```python
from build123d import *

# Parameters (mm, degrees)
SKETCH1_R           = 35
BOSS_EXTRUDE1_DEPTH = 27.6
SKETCH2_R           = 40
BOSS_EXTRUDE2_DEPTH = 2.2
BOSS_EXTRUDE3_DEPTH = 4.4
FILLET3_R           = 2
SKETCH4_R           = 6.3
CUT_EXTRUDE1_DEPTH  = 34.2
SKETCH5_R           = 2.5
CUT_EXTRUDE2_DEPTH  = 4.4


with BuildPart() as part:
    # Sketch1 → Boss-Extrude1 (new body)
    with BuildSketch(Plane(origin=(0, 0, 0), x_dir=(1, 0, 0), z_dir=(0, 1, 0))):
        with Locations(Location((0, 0, 0), (0, 0, 90))):
            Circle(SKETCH1_R)
    extrude(amount=BOSS_EXTRUDE1_DEPTH)

    # Sketch2 → Boss-Extrude2 (add)
    with BuildSketch(Plane(origin=(0, 27.6, 0), x_dir=(1, 0, 0), z_dir=(0, 1, 0))):
        with Locations(Location((0, 0, 0), (0, 0, 270))):
            Circle(SKETCH2_R)
    extrude(amount=BOSS_EXTRUDE2_DEPTH)

    # Sketch3 → Boss-Extrude3 (add)
    with BuildSketch(Plane(origin=(0, 29.8, 0), x_dir=(1, 0, 0), z_dir=(0, 1, 0))):
        with BuildLine():
            Line((-25, 5), (-17.291616466, 5))
            ThreePointArc((-17.291616466, 5), (-12.727922061, 12.727922061), (-5, 17.291616466))
            Line((-5, 17.291616466), (-5, 25))
            Line((-5, 25), (5, 25))
            Line((5, 25), (5, 17.291616466))
            ThreePointArc((5, 17.291616466), (12.727922061, 12.727922061), (17.291616466, 5))
            Line((17.291616466, 5), (25, 5))
            Line((25, 5), (25, -5))
            Line((25, -5), (17.291616466, -5))
            ThreePointArc((17.291616466, -5), (12.727922061, -12.727922061), (5, -17.291616466))
            Line((5, -17.291616466), (5, -25))
            Line((5, -25), (-5, -25))
            Line((-5, -25), (-5, -17.291616466))
            ThreePointArc((-5, -17.291616466), (-12.727922061, -12.727922061), (-17.291616466, -5))
            Line((-17.291616466, -5), (-25, -5))
            Line((-25, -5), (-25, 5))
        make_face()
    extrude(amount=BOSS_EXTRUDE3_DEPTH)

    # Fillet3
    fillet3_edges = [part.edges().sort_by_distance(p)[0] for p in [
        (-25, 32, -5),
        (-25, 32, 5),
        (-17.291616466, 32, 5),
        (-5, 32, 17.291616466),
        (-5, 32, 25),
        (5, 32, 25),
        (5, 32, 17.291616466),
        (17.291616466, 32, 5),
        (25, 32, 5),
        (25, 32, -5),
        (17.291616466, 32, -5),
        (5, 32, -17.291616466),
        (5, 32, -25),
        (-5, 32, -25),
        (-5, 32, -17.291616466),
        (-17.291616466, 32, -5),
    ]]
    fillet(fillet3_edges, radius=FILLET3_R)

    # Sketch4 → Cut-Extrude1 (cut)
    with BuildSketch(Plane(origin=(0, 34.2, 0), x_dir=(1, 0, 0), z_dir=(0, 1, 0))):
        with Locations(Location((0, 0, 0), (0, 0, 270))):
            Circle(SKETCH4_R)
    extrude(amount=-CUT_EXTRUDE1_DEPTH, mode=Mode.SUBTRACT)

    # Sketch5 → Cut-Extrude2 (cut)
    with BuildSketch(Plane(origin=(0, 34.2, 0), x_dir=(1, 0, 0), z_dir=(0, 1, 0))):
        with Locations(Location((21, 0, 0), (0, 0, 270))):
            Circle(SKETCH5_R)
        with Locations(Location((0, -21, 0), (0, 0, 270))):
            Circle(SKETCH5_R)
        with Locations(Location((-21, 0, 0), (0, 0, 270))):
            Circle(SKETCH5_R)
        with Locations(Location((0, 21, 0), (0, 0, 270))):
            Circle(SKETCH5_R)
    extrude(amount=-CUT_EXTRUDE2_DEPTH, mode=Mode.SUBTRACT)


solid = part.part
```
The model under review builds one solid part; all positions refer to its coordinate system, in mm. A direction names the side the tool comes from. Give positions to 0.01 mm unless a question says otherwise; leave off trailing zeros. Write each loop counter-clockwise with the first axis right and the second up, starting at its lowest first coordinate (ties: lowest second). Pieces come first, ordered by that corner, then holes. Notation, with made-up numbers: (-6, -15.75) - (20, -15.75) arc R19 cw to (20, 3.25) - close; hole circle Ø9 at (45.25, 26). An arc over 180 degrees is marked (long way). Answer in a Markdown table with one row per item. Add a question column.
1. We need section B-B on z = -26. Write out the cut boundary in (x, y).
2. We need section A-A on x = 0. Write out the cut boundary in (y, z).
3. Tool access review of faces 1 (the flat face through (25, 32, 0)), 2 (the cylindrical face through (24.4, 32.03, 4.43)), 3 (the cylindrical face through (-4.43, 32.03, 24.4)), 4 (the cylindrical face through (-18.52, 32.03, -0.33)), 5 (the cylindrical face through (-24.43, 32.03, -4.4)): name each direction out of +Z, -Z, +X, -X, +Y, -Y from which nothing blocks a thin tool from reaching the whole face with its end or side.
4. We need section D-D on x = -8.5. Write out the cut boundary in (y, z), then the cut area to 3 significant figures.
5. We need section C-C on y = 31.5. State how many separate pieces and enclosed holes the cut face has, then the cut area to 3 significant figures.
6. Wall thickness on line 1 along X through (y, z) = (30.9, 0); line 2 along Y through (x, z) = (-25, -23); line 3 along X through (y, z) = (13.5, 0): over which ranges is each line inside the solid? List them lowest first. Write a range as [from, to].
7. Insertion check: P1, Ø12, axis at y = 9.5, z = -23.5, coming from the -X side; P2, Ø8, axis at y = 4.5, z = -12, coming from the -X side; P3, Ø2, axis at x = 20, y = 32, coming from the +Z side; P4, Ø11.5, axis at x = 0, z = 0, coming from the -Y side. Each pin has a flat end and moves straight along its axis. Give the tip position at first contact, or say it passes through.
Ans:
| question | item | result |
|---|---|---|
| 1 | outline | (-30.4, 27.6) - (-23.43, 27.6) - (-23.43, 0) - (23.43, 0) - (23.43, 27.6) - (30.4, 27.6) - (30.4, 29.8) - (-30.4, 29.8) - close |
| 2 | outline | (0, -35) - (27.6, -35) - (27.6, -40) - (29.8, -40) - (29.8, -25) - (34.2, -25) - (34.2, -23.5) - (29.8, -23.5) - (29.8, -18.5) - (34.2, -18.5) - (34.2, -6.3) - (0, -6.3) - close; (0, 6.3) - (34.2, 6.3) - (34.2, 18.5) - (29.8, 18.5) - (29.8, 23.5) - (34.2, 23.5) - (34.2, 25) - (29.8, 25) - (29.8, 40) - (27.6, 40) - (27.6, 35) - (0, 35) - close |
| 3 | face 1 | +Z, -Z, +X, +Y |
| 3 | face 2 | +Z, +X, +Y |
| 3 | face 3 | +Z, -X, +Y |
| 3 | face 4 | +Y |
| 3 | face 5 | -Z, -X, +Y |
| 4 | outline | (0, -33.95) - (27.6, -33.95) - (27.6, -39.09) - (29.8, -39.09) - (29.8, -15.87) - (34.2, -15.87) - (34.2, 15.87) - (29.8, 15.87) - (29.8, 39.09) - (27.6, 39.09) - (27.6, 33.95) - (0, 33.95) - close |
| 4 | area | 2,190 mm^2 |
| 5 | separate pieces | 1 |
| 5 | enclosed holes | 5 |
| 5 | area | 1,100 mm^2 |
| 6 | line 1 | x = [-25, -23.5], [-18.5, -6.3], [6.3, 18.5], [23.5, 25] |
| 6 | line 2 | y = [0, 29.8] |
| 6 | line 3 | x = [-35, -6.3], [6.3, 35] |
| 7 | P1 | stops at x = -30.31 |
| 7 | P2 | stops at x = -34.07 |
| 7 | P3 | stops at z = 5 |
| 7 | P4 | passes through |
